Work out the finished part from the listing and answer in its coordinate system (mm). Coordinates: 2 decimals unless noted, no trailing zeros. Write each loop counter-clockwise with the first axis right and the second up, starting at its lowest first coordinate (ties: lowest second). Pieces come first, ordered by that corner, then holes. Notation, with made-up numbers: M -3.75,15 L 43.25,15 A29 ccw 43.25,52 Z; hole C 14,-37.5 d11. An arc over 180 degrees is marked long. Answer as CSV lines item,"result". Start each with the question number.
(1) A cutting plane is placed at D-D on y = -20.5. Give the vertices of the cut face in (x, z), then the cut area to 3 significant figures.
(2) The mould has two halves that part along Y. Classify faces 1 (the cylindrical face through (-32.03, -16.57, 7.4)), 2 (the flat face through (-35, -14, 15)), 3 (the flat face through (-34, -22.533, 7)), 4 (the cylindrical face through (-27.408, -15.742, 7.395)): released by +Y, released by -Y, zero draft, split by the parting line, or undercut.
(3) A cutting plane is placed at B-B on x = -33. Give the vertices of the cut face in (y, z), then the cut area to 3 significant figures.
(4) Find the intervals of material crossed by L1, parallel to Y at x = -33.25, z = 11.25; L2, parallel to Y at x = -35.5, z = 2; L3, parallel to X at y = -15.25, z = 5.5, in increasing order. Write a range as [from, to].
(5) A cutting plane is placed at C-C on z = 6.75. Give the vertices of the cut face in (x, y).
(6) A cutting plane is placed at A-A on y = -15.5. Give the vertices of the cut face in (x, z).
(7) Flat-ended cylindrical pins translate along their axes: P1, Ø3, axis at x = -33.78, y = -15.84, coming from the +Z side; P2, Ø5, axis at y = -10.5, z = 11.5, coming from the -X side. Find the tip coordinate at first contact, or state that the pin passes through.
from build123d import *

# Parameters (mm, degrees)
CROQUIS1_R              = 1.9
SALIENTE_EXTRUIR2_DEPTH = 15


with BuildPart() as part:
    # Croquis1 → Saliente-Extruir2 (new body)
    with BuildSketch(Plane.XY):
        with BuildLine():
            ThreePointArc((-28.784956102, -9.143234849), (-27.407440411, -15.838234849), (-28.784956102, -22.533234849))
            Line((-28.784956102, -22.533234849), (-38.784956102, -22.533234849))
            ThreePointArc((-38.784956102, -22.533234849), (-40.162471794, -15.838234849), (-38.784956102, -9.143234849))
            Line((-38.784956102, -9.143234849), (-28.784956102, -9.143234849))
        make_face()
        with Locations((-33.784956102, -15.838234849)):
            Circle(CROQUIS1_R, mode=Mode.SUBTRACT)
    extrude(amount=SALIENTE_EXTRUIR2_DEPTH)


solid = part.part
Here are the results:
1,outline,"M -39.51,0 L -28.06,0 L -28.06,15 L -39.51,15 Z"
1,area,"172 mm^2"
2,face 1,"undercut"
2,face 2,"zero draft"
2,face 3,"released by -Y"
2,face 4,"split by the parting line"
3,outline,"M -22.53,0 L -17.57,0 L -17.57,15 L -22.53,15 Z; M -14.11,0 L -9.14,0 L -9.14,15 L -14.11,15 Z"
3,area,"149 mm^2"
4,L1,"y = [-22.53, -17.66], [-14.02, -9.14]"
4,L2,"y = [-22.53, -16.66], [-15.02, -9.14]"
4,L3,"x = [-40.15, -35.59], [-31.98, -27.42]"
5,outline,"M -38.78,-22.53 L -28.78,-22.53 A16.96 ccw -28.78,-9.14 L -38.78,-9.14 A16.96 ccw Z; hole C -33.78,-15.84 d3.8"
6,outline,"M -40.16,0 L -35.65,0 L -35.65,15 L -40.16,15 Z; M -31.92,0 L -27.41,0 L -27.41,15 L -31.92,15 Z"
7,P1,"passes through"
7,P2,"stops at x = -39.92"
